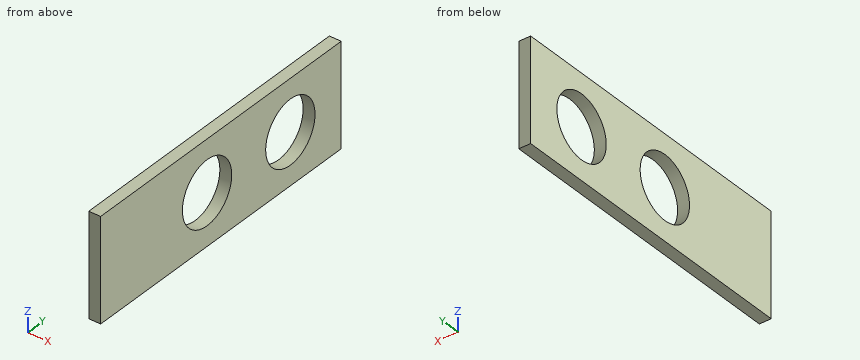
```python
from build123d import *

# Parameters (mm, degrees)
CROQUIS1_W              = 26
CROQUIS1_H              = 78
SALIENTE_EXTRUIR1_DEPTH = 3
CROQUIS2_R              = 8
CORTAR_EXTRUIR1_DEPTH   = 4


with BuildPart() as part:
    # Croquis1 → Saliente-Extruir1 (new body)
    with BuildSketch(Plane(origin=(0, 0, 0), x_dir=(0, 0, -1), z_dir=(1, 0, 0))):
        with Locations((-13, 39)):
            Rectangle(CROQUIS1_W, CROQUIS1_H)
    extrude(amount=SALIENTE_EXTRUIR1_DEPTH)

    # Croquis2 → Cortar-Extruir1 (cut, through all)
    with BuildSketch(Plane.ZY):
        with Locations((13, 61.5)):
            Circle(CROQUIS2_R)
        with Locations((13, 34.5)):
            Circle(CROQUIS2_R)
    extrude(amount=-CORTAR_EXTRUIR1_DEPTH, mode=Mode.SUBTRACT)


solid = part.part
```
Verification items for the finished model (mm, model axes). Give positions to 0.01 mm unless a question says otherwise; leave off trailing zeros. Order: outer loops, then holes, each group sorted by start corner. A loop starts at its lowest first (then second) coordinate and runs counter-clockwise, first axis right, second up. Notation, with made-up numbers: (58, 69) - (117, 69) arc R28 cw to (117, 97) - close; hole circle Ø4 at (6, 36). An arc over 180 degrees is marked (long way). Answer as CSV lines item,"result". Start each with the question number.
Item 1: Material ranges on L1, parallel to Y at x = 1.2, z = 13; L2, parallel to Y at x = 1.95, z = 11.5; L3, parallel to Z at x = 0.95, y = 55, recorded low to high.
Item 2: Section check A-A, the plane y = 61.5. Record the boundary of the cut face in (x, z).
Item 3: Gauge pin test, flat ends, axial feed: pin 1 (13 mm diameter, centred on y = 61.5, z = 13, fed in from -X); pin 2 (1 mm diameter, centred on x = 2, z = 4, fed in from -Y). Record the tip position at first contact, or that the pin passes through.
Item 4: Section check C-C, the plane x = 0.6. Record the boundary of the cut face in (y, z).
Item 5: Section check D-D, the plane y = 32. Record the boundary of the cut face in (x, z).
Item 6: Section check B-B, the plane z = 13. Record the boundary of the cut face in (x, y), plus the area to 3 significant figures.
Filled in:
1,L1,"0 to 26.5, 42.5 to 53.5, 69.5 to 78"
1,L2,"0 to 26.64, 42.36 to 53.64, 69.36 to 78"
1,L3,"0 to 8.34, 17.66 to 26"
2,outline,"(0, 0) - (3, 0) - (3, 5) - (0, 5) - close; (0, 21) - (3, 21) - (3, 26) - (0, 26) - close"
3,pin 1,"through"
3,pin 2,"y = 0"
4,outline,"(0, 0) - (78, 0) - (78, 26) - (0, 26) - close; hole circle Ø16 at (34.5, 13); hole circle Ø16 at (61.5, 13)"
5,outline,"(0, 0) - (3, 0) - (3, 5.4) - (0, 5.4) - close; (0, 20.6) - (3, 20.6) - (3, 26) - (0, 26) - close"
6,outline,"(0, 0) - (3, 0) - (3, 26.5) - (0, 26.5) - close; (0, 42.5) - (3, 42.5) - (3, 53.5) - (0, 53.5) - close; (0, 69.5) - (3, 69.5) - (3, 78) - (0, 78) - close"
6,area,"138 mm^2"
